from build123d import *

# Parameters (mm, degrees)
F0_W     = 8.61
F0_H     = 10
F1_DEPTH = 3
F4_R     = 0.5
F5_DEPTH = 25


with BuildPart() as f1:
    # F0 (on Top) → F1 (new body)
    with BuildSketch(Plane.XY):
        Rectangle(F0_W, F0_H)
    extrude(amount=-F1_DEPTH)

    # F2 (on Front) → F3 (revolve, cut)
    with BuildSketch(Plane.XZ):
        with BuildLine():
            ThreePointArc((-4.305, -0.233333), (-4.094232, -0.75461), (-3.58039, -0.982903))
            Line((-3.58039, -0.982903), (4.305, -1.25))
            Line((4.305, -1.25), (4.305, 1))
            Line((4.305, 1), (-4.305, 1))
            Line((-4.305, 1), (-4.305, -0.233333))
        make_face()
    revolve(axis=Axis((0, 0, 1), (-1, 0, 0)), mode=Mode.SUBTRACT)

    # F4 (on face) → F5 (cut)
    with BuildSketch(Plane.XY):
        with Locations((-2.305, 0)):
            Circle(F4_R)
    extrude(amount=-F5_DEPTH, mode=Mode.SUBTRACT)


solid = f1.part
For this review, take the finished solid that the model builds, in its own axes (mm). Give positions to 0.01 mm unless a question says otherwise; leave off trailing zeros. Loops run counter-clockwise (first coordinate to the right, second up) from the corner with the lowest first, then second, coordinate; pieces in that order, holes last. Notation, with made-up numbers: M 43.5,-26.5 L 59.5,-26.5 A29 ccw 59.5,-4.5 Z; hole C 3,-31.75 d6. An arc over 180 degrees is marked long. Put each result on its own line as item: value. Start each with the question number.
(1) Add section D-D, the plane x = 0. Write out the cut boundary in (y, z).
(2) Add section C-C, the plane x = 1.5. Write out the cut boundary in (y, z), then the cut area to 3 significant figures.
(3) Add section B-B, the plane y = 0. Write out the cut boundary in (x, z) (3 decimals).
(4) The part is to be moulded in two halves that separate along Y. For faces 1 (the cylindrical face through (-1.843, -0.192, -1.967)), 2 (the flat face through (-4.305, 0, -1)), 3 (the conical face through (0.42, 0.03, -1.12)), 4 (the flat face through (0, 5, -1)), say which applies: +Y half, -Y half, draft (parallel to the pull), parting line (faces both ways), or undercut.
(5) Add section A-A, the plane x = -2. Write out the cut boundary in (y, z), then the cut area to 3 significant figures.
(6) Wall thickness on L1, parallel to X at y = 0, z = -1.4 (3 decimals); L2, parallel to Y at x = -1.5, z = -0.15; L3, parallel to Y at x = -1, z = -0.55: over which ranges is each line inside the solid? List them lowest first.
Result:
1. outline: M -5,-3 L 5,-3 L 5,0 L 1.85,0 A2.1 cw -1.85,0 L -5,0 Z
2. outline: M -5,-3 L 5,-3 L 5,0 L 1.91,0 A2.15 cw -1.91,0 L -5,0 Z
2. area: 26.9 mm^2
3. outline: M -4.305,-3 L -2.805,-3 L -2.805,-1.009 L -3.58,-0.983 A0.75 cw -4.305,-0.233 Z; M -1.805,-3 L 4.305,-3 L 4.305,-1.25 L -1.805,-1.043 Z
4. face 1: undercut
4. face 2: draft
4. face 3: undercut
4. face 4: +Y half
5. outline: M -5,-3 L -0.4,-3 L -0.4,-1 A2.04 cw -1.77,0 L -5,0 Z; M 0.4,-3 L 5,-3 L 5,0 L 1.77,0 A2.04 cw 0.4,-1 Z
5. area: 25.8 mm^2
6. L1: x = -4.305 to -2.805, -1.805 to 4.305
6. L2: y = -5 to -1.7, 1.7 to 5
6. L3: y = -5 to -1.37, 1.37 to 5
